Here's how the part is built. I have some questions about the finished solid (model axes, mm). A direction names the side the tool comes from. Round coordinates to 2 decimals unless told otherwise and drop trailing zeros. Order: outer loops, then holes, each group sorted by start corner. A loop starts at its lowest first (then second) coordinate and runs counter-clockwise, first axis right, second up. Notation, with made-up numbers: (48.5, 47.5) -> (75.5, 47.5) arc R16 cw to (75.5, 72.5) -> close; hole circle Ø6 at (16.5, 27.5). An arc over 180 degrees is marked (long way). Answer in a Markdown table with one row per item.
Autodesk Inventor part; units mm, degrees
ref_plane "YZ Plane" through (0, 0, 0) normal (1, 0, 0) x (0, 1, 0)
ref_plane "XZ Plane" through (0, 0, 0) normal (0, 1, 0) x (-1, 0, 0)
ref_plane "XY Plane" through (0, 0, 0) normal (0, 0, 1) x (1, 0, 0)
sketch "Szkic1" plane through (0, 0, 0) normal (0, 1, 0) x (-1, 0, 0)
  line L0 (7.5, 5) -> (-7.5, 5)
  line L1 (-7.5, 5) -> (-7.5, -5)
  line L2 (-7.5, -5) -> (7.5, -5)
  line L3 (7.5, -5) -> (7.5, 5)
  point P0 (0, 0)
  dimension "d0" = 10
  dimension "d1" = 15
  dimension "d2" = 5
  dimension "d3" = 7.5
extrude "Wyciągnięcie proste1" add sketch "Szkic1" along normal blind 5
sketch "Szkic2" plane through (0, 5, 0) normal (0, 1, 0) x (1, 0, 0)
  line L0 (-7.5, -5) -> (7.5, -5)
  line L1 (7.5, -5) -> (7.5, 5)
  line L2 (-7.5, -5) -> (7.5, -5)
  line L3 (7.5, -5) -> (7.5, 3)
  line L4 (7.5, 3) -> (-7.5, 3)
  line L5 (-7.5, 3) -> (-7.5, -5)
  point P0 (0, 0)
  dimension "d6" = 8
extrude "Wyciągnięcie proste2" add sketch "Szkic2" along normal blind 4
sketch "Szkic3" plane through (0, 9, 0) normal (0, 1, 0) x (1, 0, 0)
  circle A0 centre (-4, -1) radius 2
  line L0 (-7.5, 3) -> (-7.5, -5)
  line L1 (7.5, 3) -> (-7.5, 3)
  circle A1 centre (4.5, -1) radius 2
  line L2 (7.5, -5) -> (7.5, 3)
  point P0 (0, 0)
  dimension "d9" = 4
  dimension "d10" = 3.5
  dimension "d11" = 4
  dimension "d12" = 3
  dimension "d13" = 4
  dimension "d14" = 4
extrude "Wyciągnięcie proste3" cut sketch "Szkic3" against normal blind 1
properties part number "Sharp"
1. Suppose I cut it at C-C on y = 5.5. Write out the boundary of the cut face in (x, z), then the cut area to 3 significant figures.
Numbers:
| item | result |
|---|---|
| outline | (-7.5, -3) -> (7.5, -3) -> (7.5, 5) -> (-7.5, 5) -> close |
| area | 120 mm2 |
2. Please list where these lines run through material, in increasing order: line 1 along X through (y, z) = (8.5, 1); line 2 along Z through (x, y) = (-4, 8.7); line 3 along Z through (x, y) = (2, 7.75).
Numbers:
| item | result |
|---|---|
| line 1 | x = -7.5 to -6, -2 to 2.5, 6.5 to 7.5 |
| line 2 | z = -3 to -1, 3 to 5 |
| line 3 | z = -3 to 5 |
3. For faces 1 (the face through (4, 8, 1)), 2 (the face through (0, 0, 0)), 3 (the face through (0, 5, -4)), which set-ups out of +Z, -Z, +X, -X, +Y, -Y let a thin tool reach every point of the face, with its end or its side?
Numbers:
| item | result |
|---|---|
| face 1 | +Y |
| face 2 | +Z, -Z, +X, -X, -Y |
| face 3 | -Z, +X, -X, +Y |
4. Suppose I cut it at B-B on z = 1. Write out the boundary of the cut face in (x, y), then the cut area to 3 significant figures.
Numbers:
| item | result |
|---|---|
| outline | (-7.5, 0) -> (7.5, 0) -> (7.5, 9) -> (6.5, 9) -> (6.5, 8) -> (2.5, 8) -> (2.5, 9) -> (-2, 9) -> (-2, 8) -> (-6, 8) -> (-6, 9) -> (-7.5, 9) -> close |
| area | 127 mm2 |
5. We'd pull the mould along Z, two halves only. Please class faces 4 (the face through (7.5, 4, 0)), 5 (the face through (2.502, 8.507, 0.912)), 6 (the face through (-4, 8, 1)), 7 (the face through (0, 7, -3)): released by +Z, released by -Z, zero draft, split by the parting line, or undercut.
Numbers:
| item | result |
|---|---|
| face 4 | zero draft |
| face 5 | undercut |
| face 6 | undercut |
| face 7 | released by -Z |
6. Suppose I cut it at A-A on x = -4. Write out the boundary of the cut face in (y, z), then the cut area to 3 significant figures.
Numbers:
| item | result |
|---|---|
| outline | (0, -5) -> (5, -5) -> (5, -3) -> (9, -3) -> (9, -1) -> (8, -1) -> (8, 3) -> (9, 3) -> (9, 5) -> (0, 5) -> close |
| area | 78.0 mm2 |
7. Suppose I cut it at D-D on z = 2.75. Write out the boundary of the cut face in (x, y), then the cut area to 3 significant figures.
Numbers:
| item | result |
|---|---|
| outline | (-7.5, 0) -> (7.5, 0) -> (7.5, 9) -> (5.47, 9) -> (5.47, 8) -> (3.53, 8) -> (3.53, 9) -> (-3.03, 9) -> (-3.03, 8) -> (-4.97, 8) -> (-4.97, 9) -> (-7.5, 9) -> close |
| area | 131 mm2 |
8. For pin 1 Ø2 at (x, z) = (-4.5, 1) entering from +Y; pin 2 Ø1 at (x, z) = (2.5, -4) entering from +Y, each with a flat end and sliding along its axis, tell me the tip position at first contact or that it passes through.
Numbers:
| item | result |
|---|---|
| pin 1 | stops at y = 8 |
| pin 2 | stops at y = 5 |
